Can you work these out from the model? Positions are in its coordinate system, mm. Face numbers are marked on the shaded views. A direction names the side the tool comes from. Give positions to 0.01 mm unless a question says otherwise; leave off trailing zeros. Order: outer loops, then holes, each group sorted by start corner. A loop starts at its lowest first (then second) coordinate and runs counter-clockwise, first axis right, second up. Notation, with made-up numbers: (-26, 89) -> (10, 89) arc R27 ccw to (10, 105) -> close; hole circle Ø6 at (-7, -14). An arc over 180 degrees is marked (long way). Answer as CSV lines item,"result".
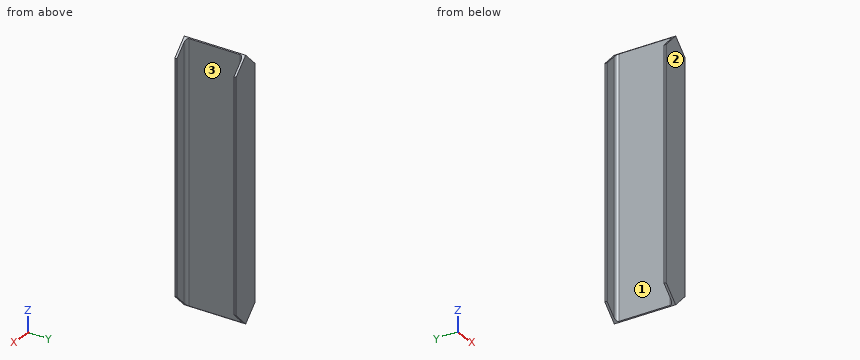
Autodesk Inventor part; units mm, degrees
ref_plane "Start Plane" through (0, 0, 0) normal (0, 0, 1) x (1, 0, 0)
ref_plane "End Plane" through (0, 0, 1500) normal (0, 0, 1) x (1, 0, 0)
ref_plane "Work Plane4" through (85, 0, -85) normal (-0.7071, 0, -0.7071) x (-0.7071, 0, 0.7071)
ref_plane "Start Plane" through (0, 0, 0) normal (0, 0, 1) x (1, 0, 0)
ref_plane "End Plane" through (0, 0, 1500) normal (0, 0, 1) x (1, 0, 0)
sketch "Sketch" plane through (0, 0, 0) normal (0, 0, 1) x (1, 0, 0)
  line L0 (-85, 167.3) -> (-22, 167.3)
  line L1 (-85, 180) -> (-85, 167.3)
  line L2 (85, 180) -> (-85, 180)
  line L3 (85, 167.3) -> (85, 180)
  line L4 (22, 167.3) -> (85, 167.3)
  line L5 (4, -149.3) -> (4, 149.3)
  line L6 (85, -167.3) -> (22, -167.3)
  line L7 (85, -180) -> (85, -167.3)
  line L8 (-85, -167.3) -> (-85, -180)
  line L9 (-22, -167.3) -> (-85, -167.3)
  line L10 (-4, 149.3) -> (-4, -149.3)
  line L11 (0, -252) -> (0, 252) construction
  line L12 (-4, -167.3) -> (4, -167.3) construction
  arc A0 (-22, -167.3) -> (-4, -149.3) centre (-22, -149.3) ccw
  arc A1 (-4, 149.3) -> (-22, 167.3) centre (-22, 149.3) ccw
  arc A2 (22, 167.3) -> (4, 149.3) centre (22, 149.3) ccw
  arc A3 (4, -149.3) -> (22, -167.3) centre (22, -149.3) ccw
  line L13 (-119, 0) -> (119, 0) construction
  line L14 (-85, -180) -> (85, -180)
  point P0 (-4, 167.3)
  point P1 (4, 167.3)
  point P2 (0, 0)
  point P3 (0, -167.3)
  point P4 (0, 0)
  dimension "d1" = 360
  dimension "d3" = 12.7
  dimension "d5" = 8
  dimension "d7" = 170
  dimension "d13" = 18
  dimension "d14" = 180
  dimension "d15" = 85
extrude "Body" add sketch "Sketch" along normal up to surface (1500 mm away) from surface at 0
sketch "Sketch3" plane through (0, 0, 0) normal (0, 0, 1) x (1, 0, 0)
  line L0 (0, 0) -> (10, 0)
ref_plane "Work Plane3" through (0, 0, 0) normal (0, -1, 0) x (1, 0, 0)
ref_plane "Work Plane4" through (85, 0, -85) normal (-0.7071, 0, -0.7071) x (-0.7071, 0, 0.7071)
split "Split1" plane through (85, 0, -85) removes the side toward (-0.7071, 0, -0.7071)
ref_plane "Work Plane5" through (-85, 0, -85) normal (0.7071, 0, -0.7071) x (-0.7071, 0, -0.7071)
split "Split2" plane through (-85, 0, -85) removes the side toward (0.7071, 0, -0.7071)
ref_plane "Work Plane6" through (-85, 0, 1585) normal (0.7071, 0, 0.7071) x (0.7071, 0, -0.7071)
split "Split3" plane through (-85, 0, 1585) removes the side toward (0.7071, 0, 0.7071)
ref_plane "Work Plane7" through (85, 0, 1585) normal (-0.7071, 0, 0.7071) x (0.7071, 0, 0.7071)
split "Split4" plane through (85, 0, 1585) removes the side toward (-0.7071, 0, 0.7071)
sketch "Sketch4" plane through (0, 0, 0) normal (0, -1, 0) x (1, 0, 0)
  line L0 (-2, 0) -> (12, 0)
  line L1 (-2, 1500) -> (12, 1500)
  dimension "d19" = 1500
equation "\"d1\" = ParH"
equation "\"d3\" = t2"
equation "\"d7\" = b"
equation "\"d13\" = R1"
equation "\"d14\" = 0.5 * d1"
equation "\"d15\" = 0.5 * d7"
equation "\"d8\" = G_L"
equation "\"b\" = 170"
equation "\"ParH\" = 360"
equation "\"R1\" = 18"
equation "\"G_L\" = d19"
equation "\"t1\" = 8"
equation "\"t2\" = 12.7"
equation "\"G_OFFSET_START\" = 0"
equation "\"G_OFFSET_END\" = 0"
properties part number "DIN 1025 - IPE 360-1500" material "Steel, Mild"
Item 1: Imagine slicing it at C-C, the plane z = 972. Please give me the cut outline in (x, y), then the cut area to 3 significant figures.
Numbers:
outline,"(-85, -180) -> (85, -180) -> (85, -167.3) -> (22, -167.3) arc R18 cw to (4, -149.3) -> (4, 149.3) arc R18 cw to (22, 167.3) -> (85, 167.3) -> (85, 180) -> (-85, 180) -> (-85, 167.3) -> (-22, 167.3) arc R18 cw to (-4, 149.3) -> (-4, -149.3) arc R18 cw to (-22, -167.3) -> (-85, -167.3) -> close"
area,"7,270 mm²"
Item 2: Imagine slicing it at A-A, the plane x = 56.5. Please give me the cut outline in (y, z).
Numbers:
outline,"(-180, 56.5) -> (-167.3, 56.5) -> (-167.3, 1443.5) -> (-180, 1443.5) -> close; (167.3, 56.5) -> (180, 56.5) -> (180, 1443.5) -> (167.3, 1443.5) -> close"
Item 3: Imagine slicing it at B-B, the plane y = -112.5. Please give me the cut outline in (x, z).
Numbers:
outline,"(-4, 4) -> (0, 0) -> (4, 4) -> (4, 1496) -> (0, 1500) -> (-4, 1496) -> close"
Item 4: For pin 1 (4 mm diameter, centred on y = 77, z = 990, fed in from -X); pin 2 (12 mm diameter, centred on y = 101, z = 975.5, fed in from +X); pin 3 (10 mm diameter, centred on x = -4, y = 80, fed in from -Z), each with a flat end and sliding along its axis, tell me the tip position at first contact or that it passes through.
Numbers:
pin 1,"stops at x = -4"
pin 2,"stops at x = 4"
pin 3,"stops at z = 0"
Item 5: For the marked faces 1, 2 and 3, which set-ups out of +Z, -Z, +X, -X, +Y, -Y let a thin tool reach every point of the face, with its end or its side?
Numbers:
face 1,"+Z, -Z, -X"
face 2,"+Z, -Z, +X, -X, -Y"
face 3,"+Z, -Z, +X"
Item 6: Please list where these lines run through material, in increasing order: line 1 along Y through (x, z) = (-62.5, 1053.5); line 2 along X through (y, z) = (16, 1341.5); line 3 along Y through (x, z) = (10.5, 954).
Numbers:
line 1,"y = -180 to -167.3, 167.3 to 180"
line 2,"x = -4 to 4"
line 3,"y = -180 to -163.15, 163.15 to 180"
